Here's how the part is built. I have some questions about the finished solid (model axes, mm). A direction names the side the tool comes from. Coordinates: 2 decimals unless noted, no trailing zeros. Write each loop counter-clockwise with the first axis right and the second up, starting at its lowest first coordinate (ties: lowest second). Pieces come first, ordered by that corner, then holes.
from build123d import *

# Parameters (mm, degrees)
SKETCH1_W           = 90.5
SKETCH1_H           = 62
BOSS_EXTRUDE2_DEPTH = 2
SKETCH5_W           = 88.5
SKETCH5_H           = 59
BOSS_EXTRUDE4_DEPTH = 1
SKETCH6_W           = 46
SKETCH6_H           = 2
BOSS_EXTRUDE5_DEPTH = 5.5
SKETCH7_W           = 15
SKETCH7_H           = 2
BOSS_EXTRUDE6_DEPTH = 10.4
SKETCH8_W           = 2
SKETCH8_H           = 22
BOSS_EXTRUDE7_DEPTH = 22.5
SKETCH9_W           = 36
SKETCH9_H           = 8
CUT_EXTRUDE3_DEPTH  = 15.9
SKETCH10_R          = 4
BOSS_EXTRUDE9_DEPTH = 17.9
SKETCH14_R          = 3
CUT_EXTRUDE7_DEPTH  = 19.9
SKETCH15_R          = 1.25
CUT_EXTRUDE8_DEPTH  = 113.625485571
SKETCH17_W          = 2
SKETCH17_H          = 40
CUT_EXTRUDE9_DEPTH  = 112.98437391


with BuildPart() as part:
    # Sketch1 → Boss-Extrude2 (new body)
    with BuildSketch(Plane(origin=(0, 0, 0), x_dir=(1, 0, 0), z_dir=(0, 1, 0))):
        with Locations((45.25, 31)):
            Rectangle(SKETCH1_W, SKETCH1_H)
    extrude(amount=BOSS_EXTRUDE2_DEPTH)

    # Sketch5 → Boss-Extrude4 (add)
    with BuildSketch(Plane(origin=(0, 2, 0), x_dir=(1, 0, 0), z_dir=(0, 1, 0))):
        with Locations((46.25, 30.5)):
            Rectangle(SKETCH5_W, SKETCH5_H)
    extrude(amount=BOSS_EXTRUDE4_DEPTH)

    # Sketch6 → Boss-Extrude5 (add)
    with BuildSketch(Plane(origin=(0, 2, 0), x_dir=(1, 0, 0), z_dir=(0, 1, 0))):
        with Locations((67.5, 1)):
            Rectangle(SKETCH6_W, SKETCH6_H)
    extrude(amount=BOSS_EXTRUDE5_DEPTH)

    # Sketch7 → Boss-Extrude6 (add)
    with BuildSketch(Plane(origin=(0, 7.5, 0), x_dir=(1, 0, 0), z_dir=(0, 1, 0))):
        with Locations((83, 1)):
            Rectangle(SKETCH7_W, SKETCH7_H)
    extrude(amount=BOSS_EXTRUDE6_DEPTH)

    # Sketch8 → Boss-Extrude7 (add)
    with BuildSketch(Plane(origin=(0, 3, 0), x_dir=(1, 0, 0), z_dir=(0, 1, 0))):
        with Locations((89.5, 11)):
            Rectangle(SKETCH8_W, SKETCH8_H)
    extrude(amount=BOSS_EXTRUDE7_DEPTH)

    # Sketch9 → Cut-Extrude3 (cut)
    with BuildSketch(Plane(origin=(0, 3, 0), x_dir=(1, 0, 0), z_dir=(0, 1, 0))):
        with Locations((20, 6)):
            Rectangle(SKETCH9_W, SKETCH9_H)
    extrude(amount=-CUT_EXTRUDE3_DEPTH, mode=Mode.SUBTRACT)

    # Sketch10 → Boss-Extrude9 (add)
    with BuildSketch(Plane(origin=(0, 3, 0), x_dir=(1, 0, 0), z_dir=(0, 1, 0))):
        with Locations(Location((28, 42, 0), (0, 0, 90))):
            Circle(SKETCH10_R)
        with Locations(Location((83, 16, 0), (0, 0, 90))):
            Circle(SKETCH10_R)
    extrude(amount=BOSS_EXTRUDE9_DEPTH)

    # Sketch14 → Cut-Extrude7 (cut)
    with BuildSketch(Plane.XZ):
        with Locations(Location((28, -42, 0), (0, 0, 270))):
            Circle(SKETCH14_R)
        with Locations(Location((83, -16, 0), (0, 0, 270))):
            Circle(SKETCH14_R)
    extrude(amount=-CUT_EXTRUDE7_DEPTH, mode=Mode.SUBTRACT)

    # Sketch15 → Cut-Extrude8 (cut, through all)
    with BuildSketch(Plane.XZ):
        with Locations(Location((28, -42, 0), (0, 0, 270))):
            Circle(SKETCH15_R)
        with Locations(Location((83, -16, 0), (0, 0, 270))):
            Circle(SKETCH15_R)
    extrude(amount=-CUT_EXTRUDE8_DEPTH, mode=Mode.SUBTRACT)

    # Sketch17 → Cut-Extrude9 (cut, through all)
    with BuildSketch(Plane(origin=(0, 3, 0), x_dir=(1, 0, 0), z_dir=(0, 1, 0))):
        with Locations((89.5, 42)):
            Rectangle(SKETCH17_W, SKETCH17_H)
    extrude(amount=-CUT_EXTRUDE9_DEPTH, mode=Mode.SUBTRACT)


solid = part.part
1. For pin 1 Ø2 at (x, z) = (81, -0.5) entering from +Y; pin 2 Ø5.5 at (x, z) = (28, -42) entering from -Y; pin 3 Ø2.5 at (x, z) = (81.5, -16) entering from +Y, each with a flat end and sliding along its axis, tell me the tip position at first contact or that it passes through.
2. On a 3-axis mill with a long thin cutter (end or side, diameter ignored), from which of +Z, -Z, +X, -X, +Y, -Y can I reach the whole of each face in a straight line? I mean faces 1 (the face through (86.905, 11.825, -15.133)), 2 (the face through (20, 2, -2)), 3 (the face through (80.07, 9.81, -15.35)), 4 (the face through (60, 7.5, -1)). Say none if no direction works.
3. I want a section at B-B (z = -5). List the corners of the cut face in (x, y) for me.
4. I want a section at A-A (y = 11.25). List the corners of the cut face in (x, z) for me, then the cut area to 3 significant figures.
5. If I drill on line 1 (X direction, y = 20.45, z = -16); line 2 (Z direction, x = 35.5, y = 2.75); line 3 (X direction, y = 5.5, z = -42), over which ranges is the centre line in solid material (lowest first)?
6. Thinking about a two-plate mould opening in X: for faces 5 (the face through (65, 7, 0)), 6 (the face through (28, 10, -39)), 7 (the face through (88.5, 2, -42)), 8 (the face through (0, 1, -31)), which applies, pulls with the +X half, pulls with the -X half, needs draft (parallel to the pull), parting line crosses it, or undercut?
7. I want a section at C-C (x = 83). List the corners of the cut face in (y, z) for me.
8. I want a section at D-D (x = 48). List the corners of the cut face in (y, z) for me, then the cut area to 3 significant figures.
Response values:
1. pin 1: stops at y = 17.9
1. pin 2: stops at y = 19.9
1. pin 3: stops at y = 20.9
2. face 1: +Y
2. face 2: +Y, -Y
2. face 3: -Y
2. face 4: +Z, -Z, -X, +Y
3. outline: (0, 0) - (2, 0) - (2, 2) - (0, 2) - close; (38, 0) - (90.5, 0) - (90.5, 25.5) - (88.5, 25.5) - (88.5, 3) - (38, 3) - close
4. outline: circle Ø8 at (28, -42); (75.5, -2) - (88.5, -2) - (88.5, -22) - (90.5, -22) - (90.5, 0) - (75.5, 0) - close; circle Ø8 at (83, -16); hole circle Ø6 at (28, -42); hole circle Ø6 at (83, -16)
4. area: 114 mm2
5. line 1: x = 79 to 81.75, 84.25 to 87, 88.5 to 90.5
5. line 2: z = -60 to -10, -2 to -1
5. line 3: x = 24 to 25, 31 to 32
6. face 5: needs draft
6. face 6: undercut
6. face 7: pulls with the +X half
6. face 8: pulls with the -X half
7. outline: (0, -62) - (2, -62) - (2, -60) - (3, -60) - (3, -20) - (20.9, -20) - (20.9, -17.25) - (19.9, -17.25) - (19.9, -19) - (0, -19) - close; (0, -13) - (19.9, -13) - (19.9, -14.75) - (20.9, -14.75) - (20.9, -12) - (3, -12) - (3, -2) - (17.9, -2) - (17.9, 0) - (0, 0) - close
8. outline: (0, -62) - (2, -62) - (2, -60) - (3, -60) - (3, -2) - (7.5, -2) - (7.5, 0) - (0, 0) - close
8. area: 193 mm2
